from build123d import *

# Parameters (mm, degrees)
SKETCH1_W           = 54
SKETCH1_H           = 30
SKETCH1_W_2         = 1.5
SKETCH1_H_2         = 17
SKETCH1_R           = 1.6
BOSS_EXTRUDE1_DEPTH = 2.4


with BuildPart() as part:
    # Sketch1 → Boss-Extrude1 (new body)
    with BuildSketch(Plane.XY):
        Rectangle(SKETCH1_W, SKETCH1_H)
        with Locations((-20.85, 0)):
            Rectangle(SKETCH1_W_2, SKETCH1_H_2, mode=Mode.SUBTRACT)
        with Locations((20.85, 0)):
            Rectangle(SKETCH1_W_2, SKETCH1_H_2, mode=Mode.SUBTRACT)
        with Locations((-6, 0)):
            Circle(SKETCH1_R, mode=Mode.SUBTRACT)
    extrude(amount=BOSS_EXTRUDE1_DEPTH)


solid = part.part
Check sheet for the modelled part. Datum: model origin and axes. Units: mm. A direction names the side the tool comes from. Give positions to 0.01 mm unless a question says otherwise; leave off trailing zeros. Loops run counter-clockwise (first coordinate to the right, second up) from the corner with the lowest first, then second, coordinate; pieces in that order, holes last. Notation, with made-up numbers: M 40,36 L 89,36 A36 ccw 89,73 Z; hole C 78,2.25 d11. An arc over 180 degrees is marked long. Answer as a JSON object with one key per item and string values. Group by question number.
Q1. Cross-section at C-C on z = 0.6. Record the cut outline in (x, y), then the cut area to 3 significant figures.
Q2. Material ranges on line 1 along X through (y, z) = (7.25, 1.9); line 2 along Y through (x, z) = (-6, 1.8), recorded low to high. Write a range as [from, to].
Q3. Cross-section at A-A on y = 0. Record the cut outline in (x, z), then the cut area to 3 significant figures.
Q4. Access from +Z, -Z, +X, -X, +Y, -Y to the whole of each face (thin tool, end or side, straight path). Record for faces 4 (the flat face through (21, 8.5, 1)), 5 (the flat face through (-27, 0, 1)).
Q5. Release check for a two-part mould opening along Y. For faces 1 (the flat face through (20.1, 0, 1)), 2 (the flat face through (0, -15, 1)), 3 (the flat face through (0, 15, 1)) record: released by +Y, released by -Y, zero draft, split by the parting line, or undercut.
Q6. Cross-section at D-D on y = -7.5. Record the cut outline in (x, z).
Q7. Cross-section at B-B on x = -6. Record the cut outline in (y, z), then the cut area to 3 significant figures.
Evaluation:
{
 "1": {"outline": "M -27,-15 L 27,-15 L 27,15 L -27,15 Z; hole M -21.6,-8.5 L -20.1,-8.5 L -20.1,8.5 L -21.6,8.5 Z; hole C -6,0 d3.2; hole M 20.1,-8.5 L 21.6,-8.5 L 21.6,8.5 L 20.1,8.5 Z", "area": "1,560 mm2"},
 "2": {"line 1": "x = [-27, -21.6], [-20.1, 20.1], [21.6, 27]", "line 2": "y = [-15, -1.6], [1.6, 15]"},
 "3": {"outline": "M -27,0 L -21.6,0 L -21.6,2.4 L -27,2.4 Z; M -20.1,0 L -7.6,0 L -7.6,2.4 L -20.1,2.4 Z; M -4.4,0 L 20.1,0 L 20.1,2.4 L -4.4,2.4 Z; M 21.6,0 L 27,0 L 27,2.4 L 21.6,2.4 Z", "area": "115 mm2"},
 "4": {"face 4": "+Z, -Z", "face 5": "+Z, -Z, -X, +Y, -Y"},
 "5": {"face 1": "undercut", "face 2": "released by -Y", "face 3": "released by +Y"},
 "6": {"outline": "M -27,0 L -21.6,0 L -21.6,2.4 L -27,2.4 Z; M -20.1,0 L 20.1,0 L 20.1,2.4 L -20.1,2.4 Z; M 21.6,0 L 27,0 L 27,2.4 L 21.6,2.4 Z"},
 "7": {"outline": "M -15,0 L -1.6,0 L -1.6,2.4 L -15,2.4 Z; M 1.6,0 L 15,0 L 15,2.4 L 1.6,2.4 Z", "area": "64.3 mm2"}
}
